Read the model definition and answer for the solid it produces. Units are mm, in the model's axes. Face numbers are marked on the shaded views. A direction names the side the tool comes from. Coordinates: 2 decimals unless noted, no trailing zeros. Write each loop counter-clockwise with the first axis right and the second up, starting at its lowest first coordinate (ties: lowest second). Pieces come first, ordered by that corner, then holes.
(1) Straight lines are drawn through the part: line 1 along X through (y, z) = (31, 3.4); line 2 along X through (y, z) = (3.1, 1.6); line 3 along Y through (x, z) = (-100.9, 3.2). For each, find the intervals that lie inside material, in ascending order.
(2) The part is cut by section B-B, the plane z = 17.5. Determine the outline of the cut face in (x, y).
(3) Which of the six approach directions +Z, -Z, +X, -X, +Y, -Y give full straight-line access (tool end or side, diameter ignored) to the marked faces 1 and 2?
(4) Given pin 1 (1 mm diameter, centred on x = -22.5, y = 52.5, fed in from +Z); pin 2 (0.6 mm diameter, centred on x = -88.5, z = 15, fed in from +Y); pin 3 (1.5 mm diameter, centred on y = 41, z = 9.5, fed in from +X); pin 4 (1.5 mm diameter, centred on x = -76, z = 6.5, fed in from -Y) (1 decimal), each flat-ended and moving along its own axis, determine where each tip first touches the part or whether it passes through.
(5) The part is cut by section C-C, the plane y = 58.9. Determine the outline of the cut face in (x, z), and give its area (3 significant figures).
(6) Determine the mould class of the marked faces 3, 4 and 5 for opening direction Y: pulls with the +Y half, pulls with the -Y half, needs draft (parallel to the pull), parting line crosses it, or undercut.
(7) The part is cut by section D-D, the plane x = -2.6. Determine the outline of the cut face in (y, z), and give its area (3 significant figures).
(8) The part is cut by section A-A, the plane x = -75.8. Determine the outline of the cut face in (y, z), and give its area (3 significant figures).
```python
from build123d import *

# Parameters (mm, degrees)
BOX_W                  = 6
BOX_H                  = 30
BOX_DEPTH              = 8
EXTRUDE001_DEPTH       = 20
CUT009_PLACEMENT_ANGLE = 180
SKETCH003_R            = 1.6
EXTRUDE003_DEPTH       = 2.5
SKETCH002_R            = 1.6
EXTRUDE002_DEPTH       = 2.5
SKETCH_R               = 1.6
EXTRUDE_DEPTH          = 10
CYLINDER007_R          = 1.6
CYLINDER007_DEPTH      = 10
CYLINDER006_R          = 1.6
CYLINDER006_DEPTH      = 10
CYLINDER005_R          = 1.6
CYLINDER005_DEPTH      = 10
CYLINDER004_R          = 1.6
CYLINDER004_DEPTH      = 10
BOX001_W               = 104
BOX001_H               = 62
BOX001_DEPTH           = 4


with BuildPart() as cube:
    # Box → Box (new body)
    with BuildSketch(Plane(origin=(-3, -15, 10.5), x_dir=(1, 0, 0), z_dir=(0, 0, 1))):
        with Locations((3, 15)):
            Rectangle(BOX_W, BOX_H)
    extrude(amount=BOX_DEPTH)


with BuildPart() as switch_holder:
    # Sketch001 → Extrude001 (new body)
    with BuildSketch(Plane.XY):
        Polygon((6.25, -9.75), (6.25, 9.75), (-6.25, 9.75), (-6.25, 3.75), (-8.25, 3.75), (-8.25, 11.75), (8.25, 11.75), (8.25, -11.75), (-8.25, -11.75), (-8.25, -6.75), (-6.25, -6.75), (-6.25, -9.75), align=None)
    extrude(amount=EXTRUDE001_DEPTH)

    # Cut009: cut Cube
    add(cube.part, mode=Mode.SUBTRACT)


with BuildPart() as switch_holder_1:
    # Cut009 placement: moved
    add(switch_holder.part.moved(Location((-95.75, 31, 4))).rotate(Axis((-95.75, 31, 4), (0, 0, 1)), CUT009_PLACEMENT_ANGLE))


with BuildPart() as nylon_nut_cutout001:
    # Sketch003 → Extrude003 (new body)
    with BuildSketch(Plane.XY):
        Polygon((3.2, 0), (1.6, 2.771281), (-1.6, 2.771281), (-3.2, 0), (-1.6, -2.771281), (1.6, -2.771281), align=None)
        Circle(SKETCH003_R, mode=Mode.SUBTRACT)
    extrude(amount=EXTRUDE003_DEPTH)


with BuildPart() as nylon_nut_cutout001_1:
    # Extrude003 placement: moved
    add(nylon_nut_cutout001.part.moved(Location((-75.8, 31, 0))))


with BuildPart() as nylon_nut_cutout:
    # Sketch002 → Extrude002 (new body)
    with BuildSketch(Plane.XY):
        Polygon((3.2, 0), (1.6, 2.771281), (-1.6, 2.771281), (-3.2, 0), (-1.6, -2.771281), (1.6, -2.771281), align=None)
        Circle(SKETCH002_R, mode=Mode.SUBTRACT)
    extrude(amount=EXTRUDE002_DEPTH)


with BuildPart() as nylon_nut_cutout_1:
    # Extrude002 placement: moved
    add(nylon_nut_cutout.part.moved(Location((-15, 31, 0))))


with BuildPart() as extrude_body:
    # Sketch → Extrude (new body)
    with BuildSketch(Plane.XY):
        with Locations((-15, 31)):
            Circle(SKETCH_R)
        with Locations((-75.8, 31)):
            Circle(SKETCH_R)
    extrude(amount=EXTRUDE_DEPTH)


with BuildPart() as mount_point003:
    # Cylinder007 → Cylinder007 (new body)
    with BuildSketch(Plane(origin=(-3.1, 58.9, 0), x_dir=(1, 0, 0), z_dir=(0, 0, 1))):
        Circle(CYLINDER007_R)
    extrude(amount=CYLINDER007_DEPTH)


with BuildPart() as mount_point002:
    # Cylinder006 → Cylinder006 (new body)
    with BuildSketch(Plane(origin=(-100.9, 58.9, 0), x_dir=(1, 0, 0), z_dir=(0, 0, 1))):
        Circle(CYLINDER006_R)
    extrude(amount=CYLINDER006_DEPTH)


with BuildPart() as mount_point001:
    # Cylinder005 → Cylinder005 (new body)
    with BuildSketch(Plane(origin=(-100.9, 3.1, 0), x_dir=(1, 0, 0), z_dir=(0, 0, 1))):
        Circle(CYLINDER005_R)
    extrude(amount=CYLINDER005_DEPTH)


with BuildPart() as mount_point:
    # Cylinder004 → Cylinder004 (new body)
    with BuildSketch(Plane(origin=(-2.6, 3.1, 0), x_dir=(1, 0, 0), z_dir=(0, 0, 1))):
        Circle(CYLINDER004_R)
    extrude(amount=CYLINDER004_DEPTH)


with BuildPart() as battery_platform:
    # Box001 → Box001 (new body)
    with BuildSketch(Plane(origin=(-104, 0, 0), x_dir=(1, 0, 0), z_dir=(0, 0, 1))):
        with Locations((52, 31)):
            Rectangle(BOX001_W, BOX001_H)
    extrude(amount=BOX001_DEPTH)

    # Cut005: cut Mount Point
    add(mount_point.part, mode=Mode.SUBTRACT)

    # Cut006: cut Mount Point001
    add(mount_point001.part, mode=Mode.SUBTRACT)

    # Cut007: cut Mount Point002
    add(mount_point002.part, mode=Mode.SUBTRACT)

    # Cut008: cut Mount Point003
    add(mount_point003.part, mode=Mode.SUBTRACT)

    # Cut: cut Extrude body
    add(extrude_body.part, mode=Mode.SUBTRACT)

    # Cut010: cut Nylon Nut Cutout
    add(nylon_nut_cutout_1.part, mode=Mode.SUBTRACT)

    # Cut011: cut Nylon Nut Cutout001
    add(nylon_nut_cutout001_1.part, mode=Mode.SUBTRACT)

    # Fusion: union Switch Holder
    add(switch_holder_1.part)


solid = battery_platform.part
```
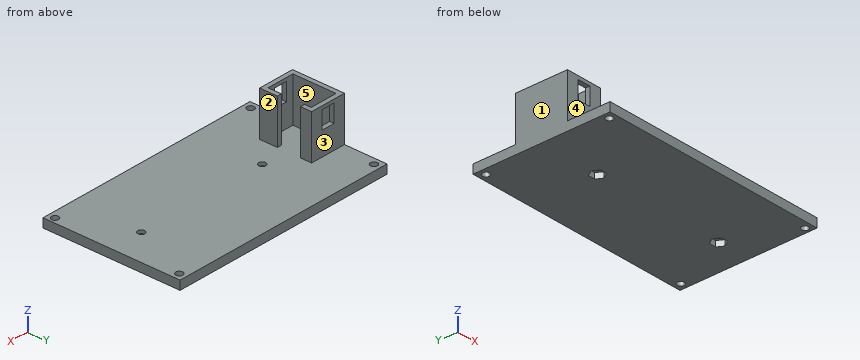
Computed:
1. line 1: x = -104 to -77.4, -74.2 to -16.6, -13.4 to 0
1. line 2: x = -104 to -102.5, -99.3 to -4.2, -1 to 0
1. line 3: y = 0 to 1.5, 4.7 to 57.3, 60.5 to 62
2. outline: (-104, 19.25) - (-98.75, 19.25) - (-98.75, 21.25) - (-102, 21.25) - (-102, 40.75) - (-98.75, 40.75) - (-98.75, 42.75) - (-104, 42.75) - close; (-92.75, 19.25) - (-87.5, 19.25) - (-87.5, 27.25) - (-89.5, 27.25) - (-89.5, 21.25) - (-92.75, 21.25) - close; (-92.75, 40.75) - (-89.5, 40.75) - (-89.5, 37.75) - (-87.5, 37.75) - (-87.5, 42.75) - (-92.75, 42.75) - close
3. face 1: +Z, -Z, -X, +Y, -Y
3. face 2: +Z, +X, +Y, -Y
4. pin 1: stops at z = 4
4. pin 2: stops at y = 42.75
4. pin 3: stops at x = -87.5
4. pin 4: passes through
5. outline: (-104, 0) - (-102.5, 0) - (-102.5, 4) - (-104, 4) - close; (-99.3, 0) - (-4.7, 0) - (-4.7, 4) - (-99.3, 4) - close; (-1.5, 0) - (0, 0) - (0, 4) - (-1.5, 4) - close
5. area: 390 mm2
6. face 3: pulls with the +Y half
6. face 4: pulls with the -Y half
6. face 5: undercut
7. outline: (0, 0) - (1.5, 0) - (1.5, 4) - (0, 4) - close; (4.7, 0) - (57.38, 0) - (57.38, 4) - (4.7, 4) - close; (60.42, 0) - (62, 0) - (62, 4) - (60.42, 4) - close
7. area: 223 mm2
8. outline: (0, 0) - (28.23, 0) - (28.23, 2.5) - (29.4, 2.5) - (29.4, 4) - (0, 4) - close; (32.6, 2.5) - (33.77, 2.5) - (33.77, 0) - (62, 0) - (62, 4) - (32.6, 4) - close
8. area: 229 mm2
